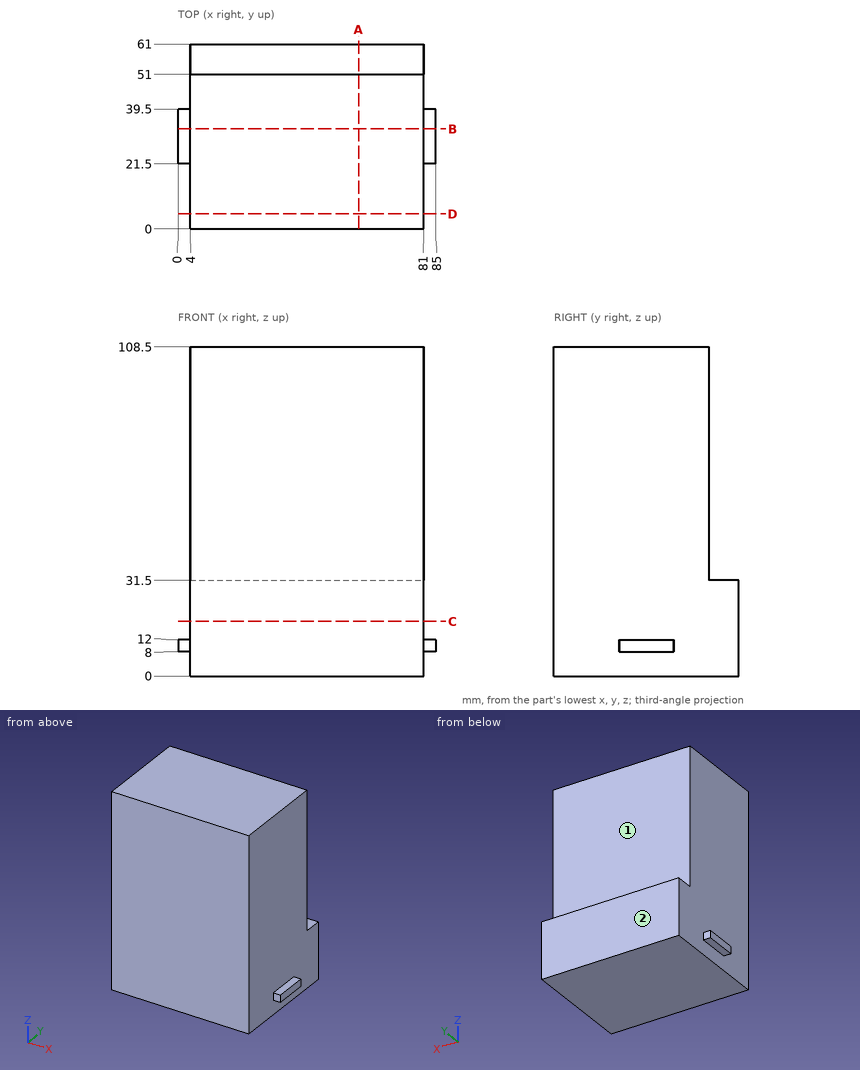
Job drawing, mm, ordinate dimensions from the low corner. One solid piece. A direction names the side the tool comes from. Give positions to 0.01 mm unless a question says otherwise; leave off trailing zeros. Write each loop counter-clockwise with the first axis right and the second up, starting at its lowest first coordinate (ties: lowest second). Pieces come first, ordered by that corner, then holes. Notation, with made-up numbers: (17.25, 47.25) - (63.25, 47.25) arc R15 ccw to (63.25, 68.25) - close; hole circle Ø3 at (48.25, 46.5). An arc over 180 degrees is marked (long way). Use one line per item in the form item = value. Start each with the question number.
1. Band-saw the part on C-C on z = 18. Write the cut outline in (x, y), plus the area to 3 significant figures.
2. Drop flat-ended pins along their axis: pin 1 Ø2 at (x, z) = (1, 10.5) entering from -Y; pin 2 Ø5 at (x, y) = (30.5, 54.5) entering from +Z; pin 3 Ø2 at (x, y) = (1.5, 26.5) entering from -Z. Give the stop position or say it passes through.
3. Probe line 1 (X direction, y = 46.5, z = 18.5); line 2 (Y direction, x = 73, z = 65); line 3 (Z direction, x = 37, y = 52). List the from-to ranges inside material, lowest first. Write a range as [from, to].
4. Band-saw the part on A-A on x = 59.5. Write the cut outline in (y, z), plus the area to 3 significant figures.
5. Band-saw the part on D-D on y = 5. Write the cut outline in (x, z).
6. 3-axis set-ups, long thin cutter, end or side, ignore diameter. For the marked faces 1 and 2: which of +Z, -Z, +X, -X, +Y, -Y reach the whole face in a straight line?
7. Band-saw the part on B-B on y = 33. Write the cut outline in (x, z), plus the area to 3 significant figures.
Conclusion:
q1.outline = (4, 0) - (81, 0) - (81, 61) - (4, 61) - close
q1.area = 4,700 mm²
q2.pin_1 = 21.5
q2.pin_2 = 31.5
q2.pin_3 = 8
q3.line_1 = [4, 81]
q3.line_2 = [0, 51]
q3.line_3 = [0, 31.5]
q4.outline = (0, 0) - (61, 0) - (61, 31.5) - (51, 31.5) - (51, 108.5) - (0, 108.5) - close
q4.area = 5,850 mm²
q5.outline = (4, 0) - (81, 0) - (81, 108.5) - (4, 108.5) - close
q6.face_1 = +Z, +X, -X, +Y
q6.face_2 = +Z, -Z, +X, -X, +Y
q7.outline = (0, 8) - (4, 8) - (4, 0) - (81, 0) - (81, 8) - (85, 8) - (85, 12) - (81, 12) - (81, 108.5) - (4, 108.5) - (4, 12) - (0, 12) - close
q7.area = 8,390 mm²
